Check sheet for the modelled part. Datum: model origin and axes. Units: mm. A direction names the side the tool comes from. Give positions to 0.01 mm unless a question says otherwise; leave off trailing zeros. Order: outer loops, then holes, each group sorted by start corner. A loop starts at its lowest first (then second) coordinate and runs counter-clockwise, first axis right, second up.
```python
from build123d import *

# Parameters (mm, degrees)
F0_R     = 14.2875
F1_DEPTH = 41.148
F0_R_2   = 6.35
F2_DEPTH = 11.176
F6_DEPTH = 3.175
F7_R     = 3.048


with BuildPart() as f1:
    # F0 (on Top) → F1 (new body)
    with BuildSketch(Plane.XY):
        with BuildLine():
            ThreePointArc((-9.966643, -23.36292), (14.00013, -21.193309), (25.4, 0))
            ThreePointArc((25.4, 0), (14.00013, 21.193309), (-9.966643, 23.36292))
            ThreePointArc((-9.966643, 23.36292), (-25.4, 0), (-9.966643, -23.36292))
        make_face()
        Circle(F0_R, mode=Mode.SUBTRACT)
    extrude(amount=F1_DEPTH)

    # F0 (on Top) → F2 (join)
    with BuildSketch(Plane.XY):
        with BuildLine():
            ThreePointArc((-9.966643, 23.36292), (14.00013, 21.193309), (25.4, 0))
            ThreePointArc((25.4, 0), (14.00013, -21.193309), (-9.966643, -23.36292))
            Line((-9.966643, -23.36292), (43.325018, -46.09719))
            ThreePointArc((43.325018, -46.09719), (61.300097, -44.469982), (69.85, -28.575))
            Line((69.85, -28.575), (69.85, 28.575))
            ThreePointArc((69.85, 28.575), (61.300097, 44.469982), (43.325018, 46.09719))
            Line((43.325018, 46.09719), (-9.966643, 23.36292))
        make_face()
        with Locations((50.8, -28.575)):
            Circle(F0_R_2, mode=Mode.SUBTRACT)
        with Locations((50.8, 28.575)):
            Circle(F0_R_2, mode=Mode.SUBTRACT)
    extrude(amount=F2_DEPTH)

    # F3 (on Front) → F4 (revolve, cut)
    with BuildSketch(Plane.XZ):
        Polygon((0, 41.148), (0, 0), (14.2875, 0), (16.256, 0), (14.224, 2.032), (14.224, 39.116), (16.256, 41.148), align=None)
    revolve(axis=Axis((0, 0, 20.574), (0, 0, -1)), mode=Mode.SUBTRACT)

    # F5 (on Front) → F6 (join, symmetric)
    with BuildSketch(Plane.XZ):
        Polygon((66.548, 11.176), (25.4, 34.932809), (21.651473, 8.582563), align=None)
    extrude(amount=F6_DEPTH, both=True)

    # F7
    f7_edges = [f1.edges().sort_by_distance(p)[0] for p in [
        (9.966643, -23.36292, 41.148),
    ]]
    fillet(f7_edges, radius=F7_R)


solid = f1.part
```
(1) Release check for a two-part mould opening along X. For faces 3 (the face through (-3.124, 14.068, 39.303)), 4 (the face through (46.26, -0.04, 22.89)), 5 (the face through (41, 3.175, 21)) record: released by +X, released by -X, zero draft, split by the parting line, or undercut.
Response values:
face 3: undercut
face 4: released by +X
face 5: zero draft
(2) Cross-section at A-A on x = 50.8. Enter the section's corners in (y, z) (3 decimals), then the cut area to 3 significant figures.
Response values:
outline: (-47.625, 0) - (-34.925, 0) - (-34.925, 11.176) - (-47.625, 11.176) - close; (-22.225, 0) - (22.225, 0) - (22.225, 11.176) - (3.175, 11.176) - (3.175, 20.268) - (-3.175, 20.268) - (-3.175, 11.176) - (-22.225, 11.176) - close; (34.925, 0) - (47.625, 0) - (47.625, 11.176) - (34.925, 11.176) - close
area: 838 mm2
(3) Cross-section at C-C on y = -33. Enter the section's corners in (x, z), then the cut area to 3 significant figures.
Response values:
outline: (12.62, 0) - (46.25, 0) - (46.25, 11.18) - (12.62, 11.18) - close; (55.35, 0) - (69.33, 0) - (69.33, 11.18) - (55.35, 11.18) - close
area: 532 mm2
(4) Gauge pin test, flat ends, axial feed: pin 1 Ø12 at (x, z) = (56.5, 17) entering from +Y; pin 2 Ø2 at (y, z) = (-6.5, 26) entering from -X; pin 3 Ø19 at (x, z) = (50, 18.5) entering from +Y (3 decimals); pin 4 Ø12 at (x, y) = (19, -37.5) entering from +Z. Record the tip position at first contact, or that the pin passes through.
Response values:
pin 1: stops at y = 47.14
pin 2: stops at x = -24.8
pin 3: stops at y = 47.625
pin 4: stops at z = 11.18
(5) Cross-section at B-B on z = 23. Enter the section's corners in (x, y) (1 decimal).
Response values:
outline: (-10, -23.4) arc R25.4 ccw to (25.2, -3.2) - (46.1, -3.2) - (46.1, 3.2) - (25.2, 3.2) arc R25.4 ccw (long way) to start; hole circle Ø28.6 at (0, 0)
(6) Material ranges on L1, parallel to Y at x = 50.8, z = 3.5 (3 decimals); L2, parallel to Y at x = 0, z = 17; L3, parallel to Y at x = 50, z = 4, recorded low to high.
Response values:
L1: y = -47.625 to -34.925, -22.225 to 22.225, 34.925 to 47.625
L2: y = -25.4 to -14.29, 14.29 to 25.4
L3: y = -47.61 to -34.87, -22.28 to 22.28, 34.87 to 47.61
(7) Set-up check for faces 1 (the face through (41, -3.175, 21)), 2 (the face through (69.85, 0, 6)): record each of +Z, -Z, +X, -X, +Y, -Y from which the full face is reachable in a straight line by a thin tool's end or side.
Response values:
face 1: +Z, +X, -Y
face 2: +Z, -Z, +X, +Y, -Y
